Geometry check sheet. Reference: the model listing, model coordinates, mm. A direction names the side the tool comes from. Coordinates: 2 decimals unless noted, no trailing zeros. Write each loop counter-clockwise with the first axis right and the second up, starting at its lowest first coordinate (ties: lowest second). Pieces come first, ordered by that corner, then holes. Notation, with made-up numbers: M -18.75,76.25 L -13.75,76.25 A21 ccw -13.75,104.25 Z; hole C 31,83 d2. An arc over 180 degrees is marked long. Write each question's results on one line, items separated by ' | '.
Autodesk Inventor part; units mm, degrees
ref_plane "YZ Plane" through (0, 0, 0) normal (1, 0, 0) x (0, 1, 0)
ref_plane "XZ Plane" through (0, 0, 0) normal (0, 1, 0) x (-1, 0, 0)
ref_plane "XY Plane" through (0, 0, 0) normal (0, 0, 1) x (1, 0, 0)
sketch "スケッチ1" plane through (0, 0, 0) normal (1, 0, 0) x (0, 1, 0)
  line L0 (0, 16.4) -> (0, 0)
  line L1 (0, 0) -> (2.4, 0)
  line L2 (2.4, 0) -> (2.4, 1.4)
  line L3 (2.4, 1.4) -> (1.3, 1.4)
  line L4 (1.3, 1.4) -> (1.3, 16.4)
  line L5 (1.3, 16.4) -> (0, 16.4)
  dimension "d1" = 1.3
  dimension "d2" = 1.4
  dimension "d3" = 2.4
  dimension "d10" = 15
revolve "回転1" add sketch "スケッチ1" angle 360 about axis through (0, 0, 16.4) along (0, 0, -1)
thread "ねじ1"
sketch "スケッチ2" plane through (0, 0, 0) normal (0, 0, -1) x (-1, 0, 0)
  line L0 (0, 0.866) -> (0.75, 0.433)
  line L1 (0.75, 0.433) -> (0.75, -0.433)
  line L2 (0.75, -0.433) -> (0, -0.866)
  line L3 (0, -0.866) -> (-0.75, -0.433)
  line L4 (-0.75, -0.433) -> (-0.75, 0.433)
  line L5 (-0.75, 0.433) -> (0, 0.866)
  line L6 (0, 2.4) -> (0, -2.4) construction
  circle A0 centre (0, 0) radius 2.4
  point P0 (0, 0)
  point P1 (0, 0)
  dimension "d7" = 1.5
extrude "押し出し1" cut sketch "スケッチ2" against normal blind 1.4 contours L0 L1 L2 L3 L4 L5
properties part number "M2_6-15" material "チタン"
Q1. Sectioned sample at A-A on y = 0. Record the cut outline in (x, z), and give its area (3 significant figures).
Geometry check:
outline: M -2.4,0 L -0.75,0 L -0.75,1.4 L 0.75,1.4 L 0.75,0 L 2.4,0 L 2.4,1.4 L 1.3,1.4 L 1.3,16.4 L -1.3,16.4 L -1.3,1.4 L -2.4,1.4 Z | area: 43.6 mm2
Q2. Scan lines: probe 1 along X at (y, z) = (-0.1, 11.25); probe 2 along Z at (x, y) = (-1.1, -2.1); probe 3 along Z at (x, y) = (0.1, 0.7). Record each from-to range of solid material in increasing order.
Geometry check:
probe 1: x = -1.3 to 1.3 | probe 2: z = 0 to 1.4 | probe 3: z = 1.4 to 16.4
Q3. Depth check by flat-ended pin: P1, Ø1, axis at x = 0.5, z = 3, coming from the -Y side; P2, Ø1.5, axis at x = -1, z = 10, coming from the +Y side. Enter the tip coordinate at first touch or a pass-through.
Geometry check:
P1: stops at y = -1.3 | P2: stops at y = 1.28
Q4. Mould release check, pull along X, two halves, no side actions. Record for faces 4 (the flat face through (0.75, 0, 1)), 5 (the cylindrical face through (-2.024, 1.29, 0.71)), 6 (the flat face through (1, -1, 0)), 7 (the flat face through (-0.75, 0, 1)): pulls with the +X half, pulls with the -X half, needs draft (parallel to the pull), parting line crosses it, or undercut.
Geometry check:
face 4: undercut | face 5: parting line crosses it | face 6: needs draft | face 7: undercut
Q5. Sectioned sample at D-D on x = -2. Record the cut outline in (y, z), and give its area (3 significant figures).
Geometry check:
outline: M -1.33,0 L 1.33,0 L 1.33,1.4 L -1.33,1.4 Z | area: 3.71 mm2
Q6. Sectioned sample at C-C on z = 14.25. Record the cut outline in (x, y), and give its area (3 significant figures).
Geometry check:
outline: C 0,0 d2.6 | area: 5.31 mm2
Q7. Sectioned sample at B-B on x = 0.15. Record the cut outline in (y, z), and give its area (3 significant figures).
Geometry check:
outline: M -2.4,0 L -0.78,0 L -0.78,1.4 L 0.78,1.4 L 0.78,0 L 2.4,0 L 2.4,1.4 L 1.29,1.4 L 1.29,16.4 L -1.29,16.4 L -1.29,1.4 L -2.4,1.4 Z | area: 43.3 mm2
Q8. Access from +Z, -Z, +X, -X, +Y, -Y to the whole of each face (thin tool, end or side, straight path). Record for faces 1 (the cylindrical face through (-1.29, -0.17, 9)), 2 (the flat face through (0, 0, 1.4)), 3 (the flat face through (0, 0, 16.4)).
Geometry check:
face 1: +Z | face 2: -Z | face 3: +Z, +X, -X, +Y, -Y
